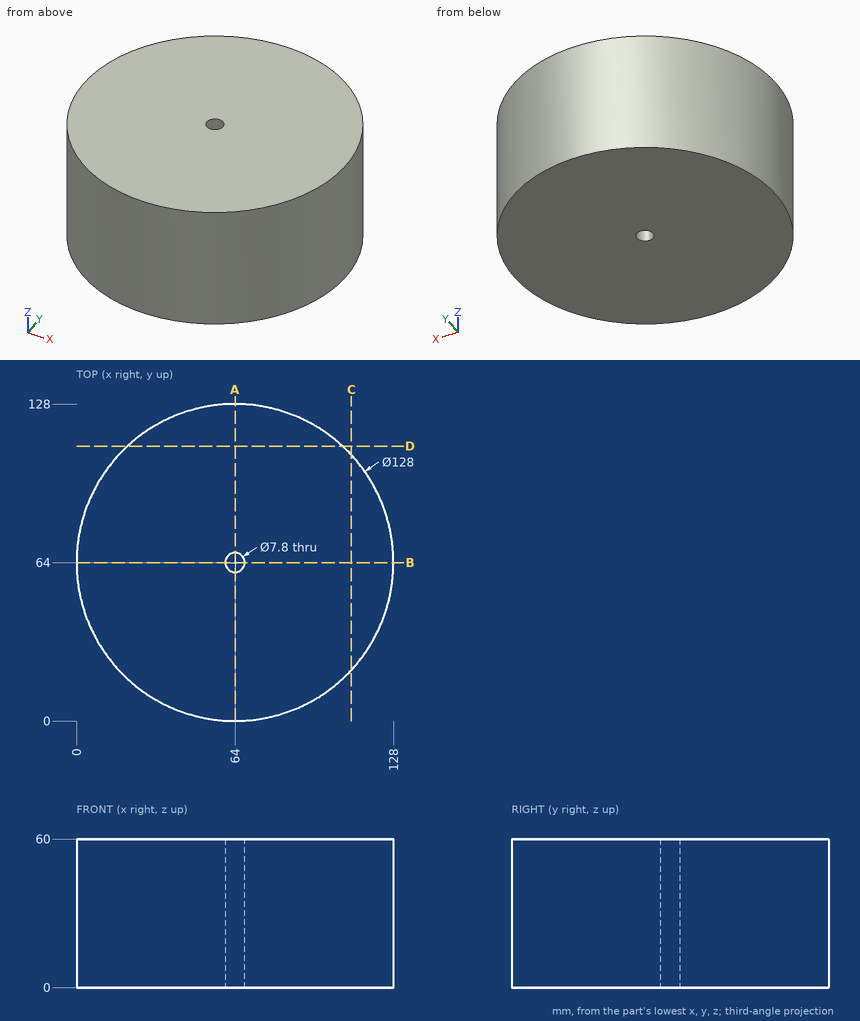
Job drawing, mm, ordinate dimensions from the low corner. One solid piece. Coordinates: 2 decimals unless noted, no trailing zeros. Order: outer loops, then holes, each group sorted by start corner. A loop starts at its lowest first (then second) coordinate and runs counter-clockwise, first axis right, second up. Notation, with made-up numbers: (23.25, 47) -> (45.25, 47) arc R12 cw to (45.25, 62) -> close; hole circle Ø11 at (16, 59.5). An arc over 180 degrees is marked (long way). Answer in a Markdown table with one row per item. Add a question column.
Q1. Band-saw the part on A-A, the plane x = 64. List the corners of the cut face in (y, z), then the cut area to 3 significant figures.
Q2. Drop flat-ended pins along their axis: pin 1 (6 mm diameter, centred on y = 33.5, z = 10, fed in from -X); pin 2 (3 mm diameter, centred on x = 74.5, z = 16.5, fed in from +Y); pin 3 (8 mm diameter, centred on x = 34, z = 40.5, fed in from +Y). Give the stop position or say it passes through.
Q3. Wall check: line 1 along Y through (x, z) = (64, 19); line 2 along Y through (x, z) = (67.5, 19.5); line 3 along Y through (x, z) = (43.5, 10). Give the ranges that are in metal, low to high. Write a range as [from, to].
Q4. Band-saw the part on C-C, the plane x = 111. List the corners of the cut face in (y, z), then the cut area to 3 significant figures.
Answers follow:
| question | item | result |
|---|---|---|
| 1 | outline | (0, 0) -> (60.1, 0) -> (60.1, 60) -> (0, 60) -> close; (67.9, 0) -> (128, 0) -> (128, 60) -> (67.9, 60) -> close |
| 1 | area | 7,210 mm^2 |
| 2 | pin 1 | x = 6.21 |
| 2 | pin 2 | y = 127.36 |
| 2 | pin 3 | y = 122.48 |
| 3 | line 1 | [0, 60.1], [67.9, 128] |
| 3 | line 2 | [0.1, 62.28], [65.72, 127.9] |
| 3 | line 3 | [3.37, 124.63] |
| 4 | outline | (20.56, 0) -> (107.44, 0) -> (107.44, 60) -> (20.56, 60) -> close |
| 4 | area | 5,210 mm^2 |
